Design review of the part shown in the three views and the two pictorial views. Dimensions are in mm from the part's minimum x, y and z. Give positions to 0.01 mm unless a question says otherwise; leave off trailing zeros. Order: outer loops, then holes, each group sorted by start corner. A loop starts at its lowest first (then second) coordinate and runs counter-clockwise, first axis right, second up. Notation, with made-up numbers: (-39, 76.25) -> (-29, 76.25) arc R30 cw to (-29, 102.25) -> close; hole circle Ø4 at (5, 45.25). An arc over 180 degrees is marked (long way). Use one line per item in the form item = value.
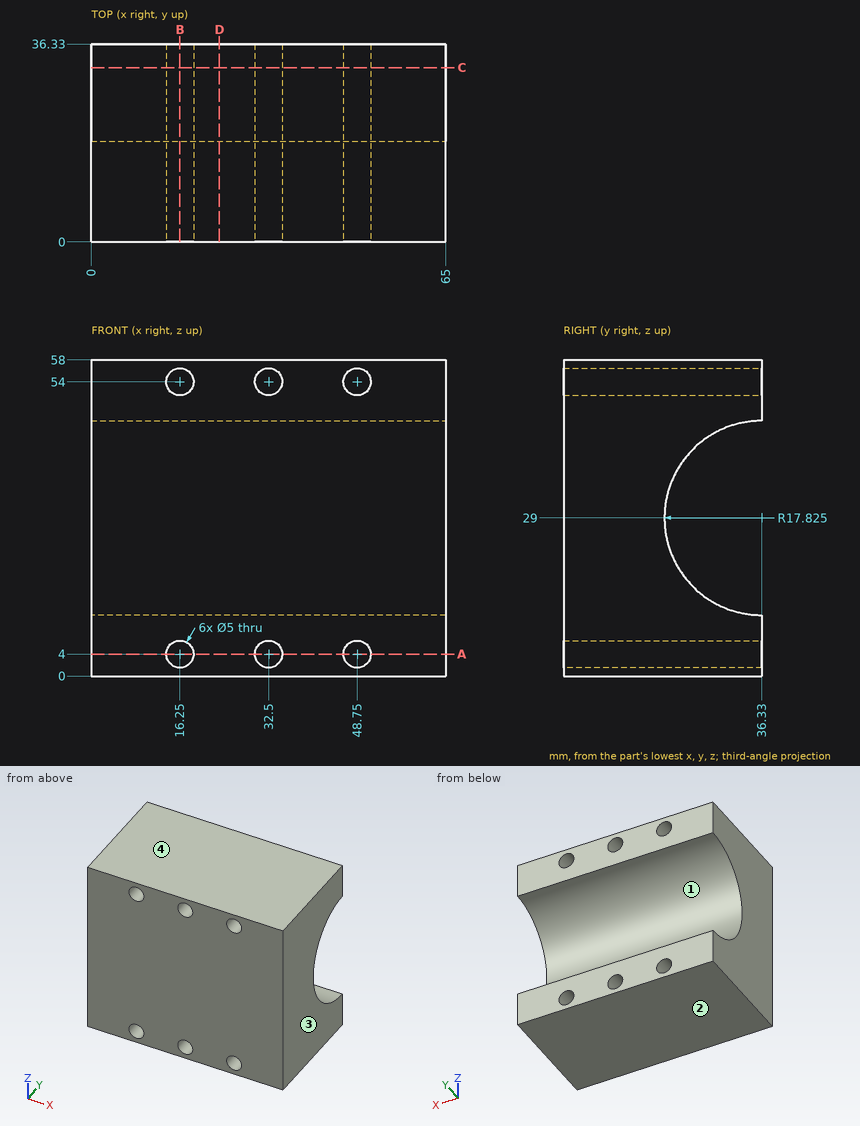
1. Add section A-A on z = 4. Give the boundary of the cut face in (x, y), then the cut area to 3 significant figures.
Values:
outline = (0, 0) -> (13.75, 0) -> (13.75, 36.33) -> (0, 36.33) -> close; (18.75, 0) -> (30, 0) -> (30, 36.33) -> (18.75, 36.33) -> close; (35, 0) -> (46.25, 0) -> (46.25, 36.33) -> (35, 36.33) -> close; (51.25, 0) -> (65, 0) -> (65, 36.33) -> (51.25, 36.33) -> close
area = 1,820 mm^2
2. For pin 1 Ø10 at (x, y) = (51.5, 25.5) entering from -Z; pin 2 Ø3 at (x, z) = (16.25, 4) entering from -Y, all flat-tipped, find the tip position at first contact; note any pin that passes through.
Values:
pin_1 = 0
pin_2 = through
3. Add section B-B on x = 16.25. Give the boundary of the cut face in (y, z) (3 decimals).
Values:
outline = (0, 0) -> (36.33, 0) -> (36.33, 1.5) -> (0, 1.5) -> close; (0, 6.5) -> (36.33, 6.5) -> (36.33, 11.175) arc R17.825 cw to (36.33, 46.825) -> (36.33, 51.5) -> (0, 51.5) -> close; (0, 56.5) -> (36.33, 56.5) -> (36.33, 58) -> (0, 58) -> close
4. Add section C-C on y = 32. Give the boundary of the cut face in (x, z).
Values:
outline = (0, 0) -> (65, 0) -> (65, 11.71) -> (0, 11.71) -> close; (0, 46.29) -> (65, 46.29) -> (65, 58) -> (0, 58) -> close; hole circle Ø5 at (16.25, 4); hole circle Ø5 at (16.25, 54); hole circle Ø5 at (32.5, 4); hole circle Ø5 at (32.5, 54); hole circle Ø5 at (48.75, 4); hole circle Ø5 at (48.75, 54)
5. For L1, parallel to X at y = 18.5, z = 4; L2, parallel to Z at x = 16, y = 9; L3, parallel to Z at x = 48, y = 26, list the stretches that pass through material, from the lowest coordinate up.
Values:
L1 = 0 to 13.75, 18.75 to 30, 35 to 46.25, 51.25 to 65
L2 = 0 to 1.51, 6.49 to 51.51, 56.49 to 58
L3 = 0 to 1.62, 6.38 to 14.47, 43.53 to 51.62, 56.38 to 58
6. Add section D-D on x = 23.5. Give the boundary of the cut face in (y, z) (3 decimals), then the cut area to 3 significant figures.
Values:
outline = (0, 0) -> (36.33, 0) -> (36.33, 11.175) arc R17.825 cw to (36.33, 46.825) -> (36.33, 58) -> (0, 58) -> close
area = 1,610 mm^2
7. The part is to be moulded in two halves that separate along Z. For the marked faces 1, 2, 3 and 4, say which applies: +Z half, -Z half, draft (parallel to the pull), parting line (faces both ways), or undercut.
Values:
face_1 = undercut
face_2 = -Z half
face_3 = draft
face_4 = +Z half
